from build123d import *

# Parameters (mm, degrees)
SKETCH_1_W          = 100
SKETCH_1_H          = 40
EXTRUDE_1_DEPTH     = 20
FILLET_2_R          = 10
CUT_EXTRUDE_1_DEPTH = 10
CUT_EXTRUDE_2_DEPTH = 55.772255751
CUT_EXTRUDE_3_DEPTH = 5
CUT_EXTRUDE_4_DEPTH = 10


with BuildPart() as part:
    # ｽｹｯﾁ1 → ﾎﾞｽ - 押し出し1 (new body)
    with BuildSketch(Plane.XY):
        Rectangle(SKETCH_1_W, SKETCH_1_H)
    extrude(amount=EXTRUDE_1_DEPTH)

    # ﾌｨﾚｯﾄ2
    fillet_2_edges = [part.edges().sort_by_distance(p)[0] for p in [
        (50, -20, 10),
        (-50, -20, 10),
        (-50, 20, 10),
        (50, 20, 10),
    ]]
    fillet(fillet_2_edges, radius=FILLET_2_R)

    # ｽｹｯﾁ2 → ｶｯﾄ - 押し出し1 (cut)
    with BuildSketch(Plane.XY.offset(20)):
        with BuildLine():
            Line((-5.1, -15.1), (5.1, -15.1))
            ThreePointArc((5.1, -15.1), (12.171067812, -12.171067812), (15.1, -5.1))
            Line((15.1, -5.1), (15.1, 5.1))
            ThreePointArc((15.1, 5.1), (12.171067812, 12.171067812), (5.1, 15.1))
            Line((5.1, 15.1), (-5.1, 15.1))
            ThreePointArc((-5.1, 15.1), (-12.171067812, 12.171067812), (-15.1, 5.1))
            Line((-15.1, 5.1), (-15.1, -5.1))
            ThreePointArc((-15.1, -5.1), (-12.171067812, -12.171067812), (-5.1, -15.1))
        make_face()
    extrude(amount=-CUT_EXTRUDE_1_DEPTH, mode=Mode.SUBTRACT)

    # ｽｹｯﾁ3 → ｶｯﾄ - 押し出し2 (cut, through all)
    with BuildSketch(Plane.XY.offset(10)):
        with BuildLine():
            Line((-4.1, -5.1), (4.1, -5.1))
            ThreePointArc((4.1, -5.1), (4.807106781, -4.807106781), (5.1, -4.1))
            Line((5.1, -4.1), (5.1, 4.1))
            ThreePointArc((5.1, 4.1), (4.807106781, 4.807106781), (4.1, 5.1))
            Line((4.1, 5.1), (-4.1, 5.1))
            ThreePointArc((-4.1, 5.1), (-4.807106781, 4.807106781), (-5.1, 4.1))
            Line((-5.1, 4.1), (-5.1, -4.1))
            ThreePointArc((-5.1, -4.1), (-4.807106781, -4.807106781), (-4.1, -5.1))
        make_face()
    extrude(amount=-CUT_EXTRUDE_2_DEPTH, mode=Mode.SUBTRACT)

    # ｽｹｯﾁ4 → ｶｯﾄ - 押し出し3 (cut)
    with BuildSketch(Plane.XY.offset(20)):
        with BuildLine():
            Line((44.1, 15.1), (35.9, 15.1))
            ThreePointArc((35.9, 15.1), (35.192893219, 14.807106781), (34.9, 14.1))
            Line((34.9, 14.1), (34.9, 5.9))
            ThreePointArc((34.9, 5.9), (35.192893219, 5.192893219), (35.9, 4.9))
            Line((35.9, 4.9), (44.1, 4.9))
            ThreePointArc((44.1, 4.9), (44.807106781, 5.192893219), (45.1, 5.9))
            Line((45.1, 5.9), (45.1, 14.1))
            ThreePointArc((45.1, 14.1), (44.807106781, 14.807106781), (44.1, 15.1))
        make_face()
        with BuildLine():
            Line((-44.1, 4.9), (-35.9, 4.9))
            ThreePointArc((-35.9, 4.9), (-35.192893219, 5.192893219), (-34.9, 5.9))
            Line((-34.9, 5.9), (-34.9, 14.1))
            ThreePointArc((-34.9, 14.1), (-35.192893219, 14.807106781), (-35.9, 15.1))
            Line((-35.9, 15.1), (-44.1, 15.1))
            ThreePointArc((-44.1, 15.1), (-44.807106781, 14.807106781), (-45.1, 14.1))
            Line((-45.1, 14.1), (-45.1, 5.9))
            ThreePointArc((-45.1, 5.9), (-44.807106781, 5.192893219), (-44.1, 4.9))
        make_face()
        with BuildLine():
            Line((45.1, -5.9), (45.1, -14.1))
            ThreePointArc((45.1, -14.1), (44.807106781, -14.807106781), (44.1, -15.1))
            Line((44.1, -15.1), (35.9, -15.1))
            ThreePointArc((35.9, -15.1), (35.192893219, -14.807106781), (34.9, -14.1))
            Line((34.9, -14.1), (34.9, -5.9))
            ThreePointArc((34.9, -5.9), (35.192893219, -5.192893219), (35.9, -4.9))
            Line((35.9, -4.9), (44.1, -4.9))
            ThreePointArc((44.1, -4.9), (44.807106781, -5.192893219), (45.1, -5.9))
        make_face()
        with BuildLine():
            Line((-44.1, -15.1), (-35.9, -15.1))
            ThreePointArc((-35.9, -15.1), (-35.192893219, -14.807106781), (-34.9, -14.1))
            Line((-34.9, -14.1), (-34.9, -5.9))
            ThreePointArc((-34.9, -5.9), (-35.192893219, -5.192893219), (-35.9, -4.9))
            Line((-35.9, -4.9), (-44.1, -4.9))
            ThreePointArc((-44.1, -4.9), (-44.807106781, -5.192893219), (-45.1, -5.9))
            Line((-45.1, -5.9), (-45.1, -14.1))
            ThreePointArc((-45.1, -14.1), (-44.807106781, -14.807106781), (-44.1, -15.1))
        make_face()
    extrude(amount=-CUT_EXTRUDE_3_DEPTH, mode=Mode.SUBTRACT)

    # ｽｹｯﾁ5 → ｶｯﾄ - 押し出し4 (cut)
    with BuildSketch(Plane(origin=(0, 0, 0), x_dir=(-1, 0, 0), z_dir=(0, 0, -1))):
        with BuildLine():
            Line((-39, -10.1), (-20.8, -10.1))
            ThreePointArc((-20.8, -10.1), (-20.092893219, -9.807106781), (-19.8, -9.1))
            Line((-19.8, -9.1), (-19.8, 9.1))
            ThreePointArc((-19.8, 9.1), (-20.092893219, 9.807106781), (-20.8, 10.1))
            Line((-20.8, 10.1), (-39, 10.1))
            ThreePointArc((-39, 10.1), (-39.707106781, 9.807106781), (-40, 9.1))
            Line((-40, 9.1), (-40, -9.1))
            ThreePointArc((-40, -9.1), (-39.707106781, -9.807106781), (-39, -10.1))
        make_face()
        with BuildLine():
            Line((20.8, -10.1), (39, -10.1))
            ThreePointArc((39, -10.1), (39.707106781, -9.807106781), (40, -9.1))
            Line((40, -9.1), (40, 9.1))
            ThreePointArc((40, 9.1), (39.707106781, 9.807106781), (39, 10.1))
            Line((39, 10.1), (20.8, 10.1))
            ThreePointArc((20.8, 10.1), (20.092893219, 9.807106781), (19.8, 9.1))
            Line((19.8, 9.1), (19.8, -9.1))
            ThreePointArc((19.8, -9.1), (20.092893219, -9.807106781), (20.8, -10.1))
        make_face()
    extrude(amount=-CUT_EXTRUDE_4_DEPTH, mode=Mode.SUBTRACT)


solid = part.part
Work out the finished part from the listing and answer in its coordinate system (mm). A direction names the side the tool comes from. Coordinates: 2 decimals unless noted, no trailing zeros. Write each loop counter-clockwise with the first axis right and the second up, starting at its lowest first coordinate (ties: lowest second). Pieces come first, ordered by that corner, then holes. Notation, with made-up numbers: (41, -12) - (55, -12) arc R10 ccw to (55, 3) - close; hole circle Ø2 at (-36, 23.5). An arc over 180 degrees is marked (long way). One line per question, with ' | ' between items.
1) Flat-ended cylindrical pins translate along their axes: P1, Ø2.5, axis at y = 11.5, z = 18, coming from the +X side; P2, Ø15, axis at x = 7, y = 6.5, coming from the +Z side; P3, Ø1, axis at x = 37, y = -0.5, coming from the -Z side. Find the tip coordinate at first contact, or state that the pin passes through.
Checks:
P1: x = 50 | P2: z = 10 | P3: z = 10
2) Find section A-A, the plane y = 2. Determine the outline of the cut face in (x, z), and give its area (3 significant figures).
Checks:
outline: (-50, 0) - (-40, 0) - (-40, 10) - (-19.8, 10) - (-19.8, 0) - (-5.1, 0) - (-5.1, 10) - (-15.1, 10) - (-15.1, 20) - (-50, 20) - close; (5.1, 0) - (19.8, 0) - (19.8, 10) - (40, 10) - (40, 0) - (50, 0) - (50, 20) - (15.1, 20) - (15.1, 10) - (5.1, 10) - close | area: 1,190 mm2
3) Find section D-D, the plane y = -11. Determine the outline of the cut face in (x, z).
Checks:
outline: (-49.95, 0) - (49.95, 0) - (49.95, 20) - (45.1, 20) - (45.1, 15) - (34.9, 15) - (34.9, 20) - (13.17, 20) - (13.17, 10) - (-13.17, 10) - (-13.17, 20) - (-34.9, 20) - (-34.9, 15) - (-45.1, 15) - (-45.1, 20) - (-49.95, 20) - close
4) Find section C-C, the plane z = 2.5. Give the number of separate pieces and of enclosed holes in the cut face, and give its area (3 significant figures).
Checks:
separate pieces: 1 | enclosed holes: 3 | area: 3,000 mm2
5) For faces 4 (the face through (12.09, -12.25, 15.07)), 5 (the face through (40, 0, 5)), 6 (the face through (-5.1, 0, 5)), determine the directions among +Z, -Z, +X, -X, +Y, -Y from which every point of the face is accessible in a straight line to the end or side of a thin tool.
Checks:
face 4: +Z | face 5: -Z | face 6: +Z, -Z
6) Find section B-B, the plane z = 13.25. Determine the outline of the cut face in (x, y).
Checks:
outline: (-50, -10) arc R10 ccw to (-40, -20) - (40, -20) arc R10 ccw to (50, -10) - (50, 10) arc R10 ccw to (40, 20) - (-40, 20) arc R10 ccw to (-50, 10) - close; hole (-15.1, -5.1) arc R10 ccw to (-5.1, -15.1) - (5.1, -15.1) arc R10 ccw to (15.1, -5.1) - (15.1, 5.1) arc R10 ccw to (5.1, 15.1) - (-5.1, 15.1) arc R10 ccw to (-15.1, 5.1) - close
7) The mould has two halves that part along X. Classify faces 1 (the face through (46.99, -17.15, 10.14)), 2 (the face through (40, 4.9, 18)), 3 (the face through (-30, -10.1, 5)): +X half, -X half, draft (parallel to the pull), parting line (faces both ways), or undercut.
Checks:
face 1: +X half | face 2: undercut | face 3: undercut
8) Consider probe 1 along X at (y, z) = (8, 9); probe 2 along Y at (x, z) = (36.5, 2); probe 3 along Y at (x, z) = (-1, 8.5). Determine where each line is inside the solid, lowest interval first. Write a range as [from, to].
Checks:
probe 1: [-50, -40], [-19.8, 19.8], [40, 50] | probe 2: [-20, -10.1], [10.1, 20] | probe 3: [-20, -5.1], [5.1, 20]
